Could you check a few things on this model? Use its own coordinates, in mm. Give positions to 0.01 mm unless a question says otherwise; leave off trailing zeros. Order: outer loops, then holes, each group sorted by start corner. A loop starts at its lowest first (then second) coordinate and runs counter-clockwise, first axis right, second up. Notation, with made-up numbers: (85, -22) - (92, -22) arc R19 cw to (92, -5) - close; hole circle Ø5 at (-11, -22.5). An arc over 180 degrees is marked (long way). Put each result on its own line as item: value.
from build123d import *

# Parameters (mm, degrees)
SKETCH_1_W          = 150
SKETCH_1_H          = 231
EXTRUDE_1_DEPTH     = 2
SKETCH_2_R          = 2.2
CUT_EXTRUDE_1_DEPTH = 2
SKETCH_3_R          = 1.6
CUT_EXTRUDE_2_DEPTH = 10
SKETCH_4_W          = 2
SKETCH_4_H          = 231
CUT_EXTRUDE_3_DEPTH = 10
SKETCH_5_W          = 2
SKETCH_5_H          = 231
CUT_EXTRUDE_4_DEPTH = 10
SKETCH_6_R          = 1.6
CUT_EXTRUDE_5_DEPTH = 10


with BuildPart() as part:
    # ｽｹｯﾁ1 → ﾎﾞｽ - 押し出し1 (new body)
    with BuildSketch(Plane.XY):
        Rectangle(SKETCH_1_W, SKETCH_1_H)
    extrude(amount=EXTRUDE_1_DEPTH)

    # ｽｹｯﾁ2 → ｶｯﾄ - 押し出し1 (cut)
    with BuildSketch(Plane.XY.offset(2)):
        with Locations((49.73, 74.5)):
            Circle(SKETCH_2_R)
        with Locations((-49.73, 74.5)):
            Circle(SKETCH_2_R)
        with Locations((0, -105.5)):
            Circle(SKETCH_2_R)
    extrude(amount=-CUT_EXTRUDE_1_DEPTH, mode=Mode.SUBTRACT)

    # ｽｹｯﾁ3 → ｶｯﾄ - 押し出し2 (cut)
    with BuildSketch(Plane.XY.offset(2)):
        with Locations((-18, -13)):
            Circle(SKETCH_3_R)
        with Locations((18, -13)):
            Circle(SKETCH_3_R)
    extrude(amount=-CUT_EXTRUDE_2_DEPTH, mode=Mode.SUBTRACT)

    # ｽｹｯﾁ4 → ｶｯﾄ - 押し出し3 (cut)
    with BuildSketch(Plane.ZY.offset(75)):
        with Locations((1, 0)):
            Rectangle(SKETCH_4_W, SKETCH_4_H)
    extrude(amount=-CUT_EXTRUDE_3_DEPTH, mode=Mode.SUBTRACT)

    # ｽｹｯﾁ5 → ｶｯﾄ - 押し出し4 (cut)
    with BuildSketch(Plane(origin=(75, 0, 0), x_dir=(0, 0, -1), z_dir=(1, 0, 0))):
        with Locations((-1, 0)):
            Rectangle(SKETCH_5_W, SKETCH_5_H)
    extrude(amount=-CUT_EXTRUDE_4_DEPTH, mode=Mode.SUBTRACT)

    # ｽｹｯﾁ6 → ｶｯﾄ - 押し出し5 (cut)
    with BuildSketch(Plane(origin=(0, 0, 0), x_dir=(-1, 0, 0), z_dir=(0, 0, -1))):
        with Locations((-12.5, 105.5)):
            Circle(SKETCH_6_R)
        with Locations((12.5, 105.5)):
            Circle(SKETCH_6_R)
    extrude(amount=-CUT_EXTRUDE_5_DEPTH, mode=Mode.SUBTRACT)


solid = part.part
1) Suppose I cut it at A-A, the plane y = -105.5. List the corners of the cut face in (x, z) for me, and give its area (3 significant figures).
Filled in:
outline: (-65, 0) - (-2.2, 0) - (-2.2, 2) - (-65, 2) - close; (2.2, 0) - (65, 0) - (65, 2) - (2.2, 2) - close
area: 251 mm^2
2) We'd pull the mould along X, two halves only. Please class faces 1 (the cylindrical face through (1.183, -103.645, 1.014)), 2 (the flat face through (-1, 2, 0)): pulls with the +X half, pulls with the -X half, needs draft (parallel to the pull), parting line crosses it, or undercut.
Filled in:
face 1: undercut
face 2: needs draft
3) If I drill on line 1 (X direction, y = 105.5, z = 0.7); line 2 (Y direction, x = 0, z = 1.4); line 3 (Y direction, x = 18, z = 1.6), over which ranges is the centre line in solid material (lowest first)? Write a range as [from, to].
Filled in:
line 1: x = [-65, -14.1], [-10.9, 10.9], [14.1, 65]
line 2: y = [-115.5, -107.7], [-103.3, 115.5]
line 3: y = [-115.5, -14.6], [-11.4, 115.5]
4) Suppose I cut it at B-B, the plane x = -49.73. List the corners of the cut face in (y, z) for me.
Filled in:
outline: (-115.5, 0) - (72.3, 0) - (72.3, 2) - (-115.5, 2) - close; (76.7, 0) - (115.5, 0) - (115.5, 2) - (76.7, 2) - close
